from build123d import *

# Parameters (mm, degrees)
CHAMFER_1_SIZE      = 0.3
CHAMFER_1_SIZE2     = 0.519615242
FILLET_1_R          = 0.4
FILLET_2_SIZE       = 0.5
FILLET_2_SIZE_2     = 0.8
CUT_EXTRUDE_1_DEPTH = 2


with BuildPart() as part:
    # 草图2 → 旋转1 (revolve)
    with BuildSketch(Plane(origin=(0, 0, 0), x_dir=(0, 0, -1), z_dir=(1, 0, 0)), mode=Mode.PRIVATE) as revolve_1_sk:
        Polygon((-7, 0), (-7, 3.4), (-3, 3.4), (-3, 2), (7, 2), (7, 0), align=None)
    revolve(revolve_1_sk.sketch.rotate(Axis((0, 0, -7), (0, 0, 1)), 90), axis=Axis((0, 0, -7), (0, 0, 1)))

    # 倒角1
    chamfer_1_edges = [part.edges().sort_by_distance(p)[0] for p in [
        (2, 0, -7),
    ]]
    chamfer_1_side = [part.faces().sort_by_distance(p)[0] for p in [
        (2, 0, -2),
    ]]
    chamfer(chamfer_1_edges, length=CHAMFER_1_SIZE, length2=CHAMFER_1_SIZE2, reference=chamfer_1_side[0])

    # 圆角1
    fillet_1_edges = [part.edges().sort_by_distance(p)[0] for p in [
        (3.4, 0, 3),
    ]]
    fillet(fillet_1_edges, radius=FILLET_1_R)

    # 圆角2
    # an asymmetric fillet: 0.8, 0.5 mm, written as the material it takes off along each edge
    with BuildSketch(Plane(origin=(0, 0, 7), x_dir=(-1, 0, 0), z_dir=(0, 1, 0))) as fillet_2_piece_1:
        with BuildLine():
            Bezier((3.4, -FILLET_2_SIZE), (3.4, 0), (3.4 - FILLET_2_SIZE_2, 0), weights=[1, 0.707106781, 1])
            Line((3.4 - FILLET_2_SIZE_2, 0), (3.4, 0))
            Line((3.4, 0), (3.4, -FILLET_2_SIZE))
        make_face()
    revolve(axis=Axis((0, 0, 7), (0, 0, 1)), mode=Mode.SUBTRACT)

    # 草图3 → 切除-拉伸1 (cut)
    with BuildSketch(Plane.XY.offset(7)):
        Polygon((0, 1.732050808), (-1.5, 0.866025404), (-1.5, -0.866025404), (0, -1.732050808), (1.5, -0.866025404), (1.5, 0.866025404), align=None)
    extrude(amount=-CUT_EXTRUDE_1_DEPTH, mode=Mode.SUBTRACT)


solid = part.part
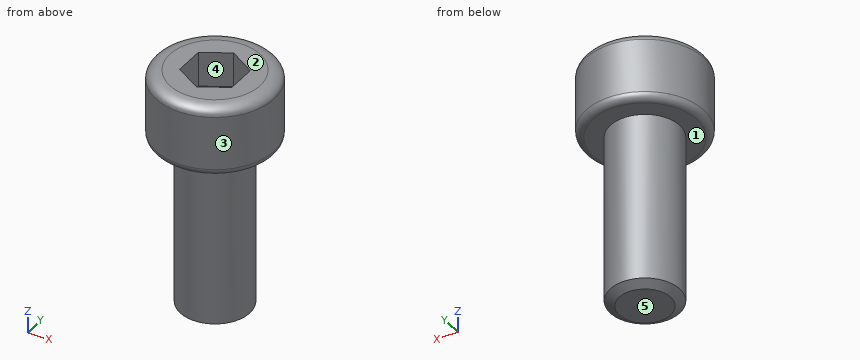
Geometry: final body of the model. Coordinates: model frame, mm. Face numbers are marked on the shaded views. A direction names the side the tool comes from. Round coordinates to 2 decimals unless told otherwise and drop trailing zeros. Loops run counter-clockwise (first coordinate to the right, second up) from the corner with the lowest first, then second, coordinate; pieces in that order, holes last. Notation, with made-up numbers: M 43.5,37.5 L 81.5,37.5 A29 cw 81.5,74.5 Z; hole C -17.75,-17 d10. An arc over 180 degrees is marked long. One line per question, with ' | ' between items.
(1) Cut plane A-A on z = 5.5. Return the cut outline in (x, y), plus the area to 3 significant figures.
Check result:
outline: C 0,0 d6.8; hole M -1.5,-0.87 L 0,-1.73 L 1.5,-0.87 L 1.5,0.87 L 0,1.73 L -1.5,0.87 Z | area: 28.5 mm2
(2) Access query for the marked faces 1 and 2. Directions: +Z, -Z, +X, -X, +Y, -Y. A direction counts if a zero-diameter tool reaches every point of the face in a straight line with its end or side. Return the directions, or none.
Check result:
face 1: -Z | face 2: +Z, +X, -X, +Y, -Y
(3) Cut plane B-B on z = -5. Return the cut outline in (x, y).
Check result:
outline: C 0,0 d4
(4) Material intervals for line 1 along X through (y, z) = (1, 1.5); line 2 along Z through (x, y) = (-2.25, 1.25), sorted ascending. Write a range as from..to.
Check result:
line 1: x = -1.73..1.73 | line 2: z = 3..7
(5) Contact query for flat-ended pins moving along their axis: P1, Ø0.9, axis at x = 0, y = 0, coming from the +Z side; P2, Ø3, axis at y = -2.5, z = 2, coming from the +X side; P3, Ø1.5, axis at x = -2, z = 3.5, coming from the +Y side. Output: stop coordinate, or through.
Check result:
P1: stops at z = 5 | P2: stops at x = 2.94 | P3: stops at y = 3.16
(6) Pull-direction query (X, two-part tool) for the marked faces 3, 4 and 5; classes: +X half, -X half, draft (parallel to the pull), parting line (faces both ways), or undercut.
Check result:
face 3: parting line | face 4: undercut | face 5: draft
